Design review of the part built by this model. Coordinates are the model's own, in mm. Give positions to 0.01 mm unless a question says otherwise; leave off trailing zeros. Order: outer loops, then holes, each group sorted by start corner. A loop starts at its lowest first (then second) coordinate and runs counter-clockwise, first axis right, second up. Notation, with made-up numbers: M -19.5,-29.75 L 20.5,-29.75 A37 ccw 20.5,8.25 Z; hole C 75.25,35.25 d1. An arc over 180 degrees is marked long. Answer as a JSON object with one key per item and string values.
from build123d import *

# Parameters (mm, degrees)
SKETCH3_R           = 14.7701
SKETCH3_R_2         = 13.3223
BOSS_EXTRUDE1_DEPTH = 1219.2
SKETCH6_R           = 6.35
SKETCH6_R_2         = 3.175
CUT_EXTRUDE2_DEPTH  = 1220.647251983


with BuildPart() as part:
    # Sketch3 → Boss-Extrude1 (new body)
    with BuildSketch(Plane(origin=(0, 0, 0), x_dir=(0, 0, -1), z_dir=(1, 0, 0))):
        with Locations(Location((0, 0, 0), (0, 0, 180))):
            Circle(SKETCH3_R)
        with Locations(Location((0, 0, 0), (0, 0, 180))):
            Circle(SKETCH3_R_2, mode=Mode.SUBTRACT)
    extrude(amount=BOSS_EXTRUDE1_DEPTH)

    # Sketch6 → Cut-Extrude2 (cut, through all)
    with BuildSketch(Plane(origin=(0, -14.7701, 0), x_dir=(-1, 0, 0), z_dir=(0, -1, 0))):
        with Locations(Location((-1117.6, 0, 0), (0, 0, 90))):
            Circle(SKETCH6_R)
        with Locations(Location((-12.7, 0, 0), (0, 0, 90))):
            Circle(SKETCH6_R_2)
    extrude(amount=-CUT_EXTRUDE2_DEPTH, mode=Mode.SUBTRACT)


solid = part.part
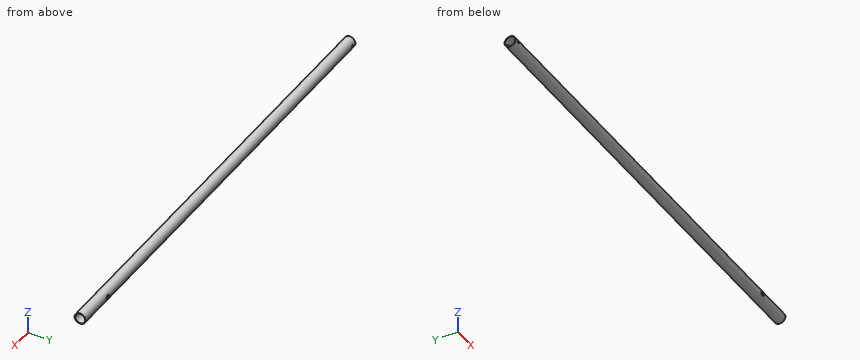
(1) We need section B-B (x = 313). Write out the cut boundary in (y, z), plus the area to 3 significant figures.
Checked values:
{"outline": "C 0,0 d29.54; hole C 0,0 d26.64", "area": "128 mm^2"}
(2) Insertion check: pin 1 (1 mm diameter, centred on x = 834, z = -11, fed in from +Y); pin 2 (8 mm diameter, centred on x = 828, y = 9, fed in from -Z); pin 3 (7.5 mm diameter, centred on x = 1117.6, z = 0, fed in from -Y); pin 4 (4 mm diameter, centred on x = 683.5, y = 8.5, fed in from -Z). Each pin has a flat end and moves straight along its axis. Give the tip position at first contact, or say it passes through.
Checked values:
{"pin 1": "stops at y = 10.39", "pin 2": "stops at z = -13.9", "pin 3": "passes through", "pin 4": "stops at z = -13.26"}
(3) We need section A-A (y = 6). Write out the cut boundary in (x, z).
Checked values:
{"outline": "M 0,-13.5 L 1219.2,-13.5 L 1219.2,-11.89 L 0,-11.89 Z; M 0,11.89 L 1219.2,11.89 L 1219.2,13.5 L 0,13.5 Z"}
(4) To check wall thickness, follow L1, parallel to X at y = -14.4, z = 0 (3 decimals); L2, parallel to Y at x = 233, z = -0.75; L3, parallel to Z at x = 368, y = 12.25. State the ranges of each line that lie inside material, in increasing order. Write a range as from..to.
Checked values:
{"L1": "x = 0..9.525, 15.875..1111.25, 1123.95..1219.2", "L2": "y = -14.75..-13.3, 13.3..14.75", "L3": "z = -8.25..-5.24, 5.24..8.25"}
